Part model, mm, in its own coordinate system. A direction names the side the tool comes from. Give positions to 0.01 mm unless a question says otherwise; leave off trailing zeros. Write each loop counter-clockwise with the first axis right and the second up, starting at its lowest first coordinate (ties: lowest second). Pieces come first, ordered by that corner, then holes.
```python
from build123d import *


with BuildPart() as part:
    # Sketch1 → Revolve1 (revolve)
    with BuildSketch(Plane.XY, mode=Mode.PRIVATE) as revolve1_sk:
        Polygon((4.005, 0), (4.005, 11), (5.5, 11), (7.5, 9), (7.5, 8), (5.995, 8), (5.995, 0), align=None)
    revolve(revolve1_sk.sketch.rotate(Axis((0, 0, 0), (0, 1, 0)), 90), axis=Axis((0, 0, 0), (0, 1, 0)))


solid = part.part
```
1) Saw through at B-B, the plane z = 0. Write the cut outline in (x, y) (3 decimals).
Answers follow:
outline: (-7.5, 8) - (-5.995, 8) - (-5.995, 0) - (-4.005, 0) - (-4.005, 11) - (-5.5, 11) - (-7.5, 9) - close; (4.005, 0) - (5.995, 0) - (5.995, 8) - (7.5, 8) - (7.5, 9) - (5.5, 11) - (4.005, 11) - close
2) Saw through at C-C, the plane y = 1.25. Write the cut outline in (x, z) (3 decimals), then the cut area to 3 significant figures.
Answers follow:
outline: circle Ø11.99 at (0, 0); hole circle Ø8.01 at (0, 0)
area: 62.5 mm2
3) Saw through at D-D, the plane y = 8.5. Write the cut outline in (x, z) (3 decimals), then the cut area to 3 significant figures.
Answers follow:
outline: circle Ø15 at (0, 0); hole circle Ø8.01 at (0, 0)
area: 126 mm2
4) Two-plate mould, pull along Y, no slides. Class faces 3 (the face through (-1.2, 5.58, -3.82)), 4 (the face through (-1.42, 0, -3.91)), 5 (the face through (5.491, 10.875, 1.219)): +Y half, -Y half, draft (parallel to the pull), parting line (faces both ways), or undercut.
Answers follow:
face 3: draft
face 4: -Y half
face 5: +Y half
5) Saw through at A-A, the plane x = 0. Write the cut outline in (y, z) (3 decimals).
Answers follow:
outline: (0, -5.995) - (8, -5.995) - (8, -7.5) - (9, -7.5) - (11, -5.5) - (11, -4.005) - (0, -4.005) - close; (0, 4.005) - (11, 4.005) - (11, 5.5) - (9, 7.5) - (8, 7.5) - (8, 5.995) - (0, 5.995) - close
6) 3-axis set-ups, long thin cutter, end or side, ignore diameter. For faces 1 (the face through (2, 8, 6)), 2 (the face through (2, 11, -4)): which of +Z, -Z, +X, -X, +Y, -Y reach the whole face in a straight line?
Answers follow:
face 1: -Y
face 2: +Z, -Z, +X, -X, +Y
7) Wall check: L1, parallel to X at y = 5.5, z = 0 (3 decimals); L2, parallel to X at y = 8.5, z = 0 (3 decimals); L3, parallel to Z at x = 1.5, y = 2. Give the ranges that are in metal, low to high.
Answers follow:
L1: x = -5.995 to -4.005, 4.005 to 5.995
L2: x = -7.5 to -4.005, 4.005 to 7.5
L3: z = -5.8 to -3.71, 3.71 to 5.8
8) Pin check, flat tips, straight feed: pin 1 Ø6 at (y, z) = (4.5, 0.5) entering from +X (3 decimals); pin 2 Ø5 at (y, z) = (1.5, 2) entering from -X (3 decimals); pin 3 Ø6 at (y, z) = (8.5, 5) entering from +X. Stop position of each tip, or through.
Answers follow:
pin 1: stops at x = 5.995
pin 2: stops at x = -5.995
pin 3: stops at x = 7.23
